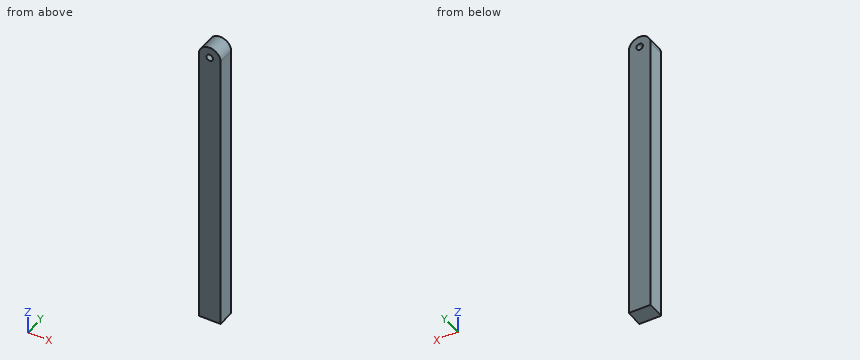
Autodesk Inventor part; units mm, degrees
ref_plane "YZ Plane" through (0, 0, 0) normal (1, 0, 0) x (0, 1, 0)
ref_plane "XZ Plane" through (0, 0, 0) normal (0, 1, 0) x (-1, 0, 0)
ref_plane "XY Plane" through (0, 0, 0) normal (0, 0, 1) x (1, 0, 0)
sketch "Sketch1" plane through (0, 0, 0) normal (0, 1, 0) x (-1, 0, 0)
  line L0 (0, 0) -> (0, -244.795) construction
  line L1 (-5, 0) -> (-5, -244.795)
  line L2 (5, -244.795) -> (5, 0)
  arc A0 (5, 0) -> (-5, 0) centre (0, 0) ccw
  arc A1 (-5, -244.795) -> (5, -244.795) centre (0, -244.795) ccw
  circle A2 centre (0, 0) radius 1.5
  circle A3 centre (0, -244.795) radius 1.5
  point P0 (0, -122.3975)
  dimension "d0" = 244.795
  dimension "d1" = 10
  dimension "d2" = 3
  dimension "d3" = 3
extrude "Extrusion1" add sketch "Sketch1" along normal blind 8
sketch "Sketch2" plane through (0, 8, 0) normal (0, 1, 0) x (1, 0, 0)
  arc A0 (5, 244.795) -> (-5, 244.795) centre (0, 244.795) ccw
  line L0 (-5, 244.795) -> (-5, 0)
  arc A1 (-5, 0) -> (5, 0) centre (0, 0) ccw
  line L1 (5, 0) -> (5, 244.795)
  circle A2 centre (0, 244.795) radius 1.5
  circle A3 centre (0, 0) radius 1.5
  circle A4 centre (0, 244.795) radius 5
  point P0 (-5, 244.795)
  dimension "d12" = 10
extrude "Extrusion2" add sketch "Sketch2" along normal blind 12 contours A4 A0
sketch "Sketch3" plane through (0, 0, 0) normal (0, -1, 0) x (1, 0, 0)
  arc A0 (-5, -244.795) -> (5, -244.795) centre (0, -244.795) ccw
  line L0 (5, 0) -> (5, -244.795)
  arc A1 (5, 0) -> (-5, 0) centre (0, 0) ccw
  line L1 (-5, -244.795) -> (-5, 0)
  circle A2 centre (0, -244.795) radius 1.5
  circle A3 centre (0, 0) radius 1.5
sketch "Sketch4" plane through (0, 20, -244.795) normal (0, 1, 0) x (1, 0, 0)
  circle A0 centre (0, 0) radius 10
  point P0 (0, -244.795)
  dimension "d15" = 20
extrude "Extrusion3" add sketch "Sketch4" against normal blind 3
sketch "Sketch5" plane through (0, 0, 0) normal (0, -1, 0) x (1, 0, 0)
  line L0 (23.0807, 11.4027) -> (-31.8332, 11.4027)
  line L1 (-31.8332, 11.4027) -> (-31.8332, -131.2308)
  line L2 (-31.8332, -131.2308) -> (23.0807, -131.2308)
  line L3 (23.0807, -131.2308) -> (23.0807, 11.4027)
  line L4 (55.5298, 55.2625) -> (-102.4368, 55.2625)
  line L5 (-102.4368, 55.2625) -> (-102.4368, -369.4288)
  line L6 (-102.4368, -369.4288) -> (55.5298, -369.4288)
  line L7 (55.5298, -369.4288) -> (55.5298, 55.2625)
  point P0 (0, 0)
extrude "Extrusion4" cut sketch "Sketch5" against normal blind 100
properties part number "Part_12_p1"
Verification items for the finished model (mm, model axes). Round coordinates to 2 decimals unless told otherwise and drop trailing zeros. Loops run counter-clockwise (first coordinate to the right, second up) from the corner with the lowest first, then second, coordinate; pieces in that order, holes last. Notation, with made-up numbers: (34, -24) -> (88, -24) arc R34 ccw to (88, 12) -> close; hole circle Ø2 at (31, 41.25). An arc over 180 degrees is marked (long way). Answer as a JSON object with one key per item and string values.
Q1. Scan lines: line 1 (Z direction, x = -0.25, y = 4.5); line 2 (Z direction, x = 0.5, y = 1.5); line 3 (Z direction, x = 1.75, y = 2.75). Record each from-to range of solid material in increasing order. Write a range as from..to.
Data:
{"line 1": "z = -131.23..-1.48, 1.48..4.99", "line 2": "z = -131.23..-1.41, 1.41..4.97", "line 3": "z = -131.23..4.68"}
Q2. Go/stop test with a flat-tipped pin: P1, Ø1, axis at x = -2.5, y = 5.5, coming from the +Z side. Record where the tip stops, or that it passes through.
Data:
{"P1": "stops at z = 4.58"}
Q3. Section check A-A (x = 0). Record the boundary of the cut face in (y, z).
Data:
{"outline": "(0, -131.23) -> (8, -131.23) -> (8, -1.5) -> (0, -1.5) -> close; (0, 1.5) -> (8, 1.5) -> (8, 5) -> (0, 5) -> close"}
